The model under review builds one solid part; all positions refer to its coordinate system, in mm. A direction names the side the tool comes from. Round coordinates to 2 decimals unless told otherwise and drop trailing zeros. Order: outer loops, then holes, each group sorted by start corner. A loop starts at its lowest first (then second) coordinate and runs counter-clockwise, first axis right, second up. Notation, with made-up numbers: M -31,43 L 9,43 A27 ccw 9,78 Z; hole C -1.5,71 d11. An arc over 180 degrees is marked long. Answer as CSV lines item,"result". Start each with the question number.
Autodesk Inventor part; units mm, degrees
ref_plane "YZ Plane" through (0, 0, 0) normal (1, 0, 0) x (0, 1, 0)
ref_plane "XZ Plane" through (0, 0, 0) normal (0, 1, 0) x (-1, 0, 0)
ref_plane "XY Plane" through (0, 0, 0) normal (0, 0, 1) x (1, 0, 0)
sketch "Sketch1" plane through (0, 0, 0) normal (0, 1, 0) x (-1, 0, 0)
  line L0 (40, 20) -> (-40, 20) construction
  line L1 (-40, 20) -> (-40, -20) construction
  line L2 (-40, -20) -> (40, -20) construction
  line L3 (40, -20) -> (40, 20) construction
  line L4 (-40, 20) -> (40, -20) construction
  line L5 (0, 20) -> (0, -20) construction
  line L6 (-45, -25) -> (-45, 0)
  line L7 (-20, -25) -> (-45, -25)
  arc A0 (69.6915, -55.359) -> (90.0175, -26.0792) centre (75.7771, -37.8885) ccw
  circle A1 centre (75.7771, -37.8885) radius 8.5
  line L8 (69.6915, -55.359) -> (-15.0657, -25.8348)
  arc A2 (-15.0657, -25.8348) -> (-20, -25) centre (-20, -40) ccw
  arc A3 (90.0175, -26.0792) -> (69.6915, -55.359) centre (75.7771, -37.8885) ccw construction
  line L9 (-45, 0) -> (-45, 25)
  line L10 (-45, 25) -> (46.484, 25)
  line L11 (40, 0) -> (45, 0) construction
  line L12 (0, 20) -> (0, 25) construction
  line L13 (-40, 0) -> (-45, 0) construction
  line L14 (47.6585, 25) -> (48.4083, 24.0959) construction
  arc A4 (48.4083, 24.0959) -> (46.484, 25) centre (46.484, 22.5) ccw
  arc A5 (46.484, 25) -> (48.4083, 24.0959) centre (46.484, 22.5) ccw construction
  line L15 (48.4083, 24.0959) -> (90.0175, -26.0792)
  line L16 (46.484, 25) -> (47.6585, 25) construction
  point P0 (0, 0)
  point P1 (0, 0)
  point P2 (0, 0)
  dimension "d2" = 80
  dimension "d3" = 40
  dimension "d29" = 5
  dimension "d30" = 17
  dimension "d31" = 10
  dimension "d32" = 40
  dimension "d34" = 5
  dimension "d35" = 15
  dimension "d36" = 25
  dimension "d38" = 5
  dimension "d41" = 66.3579
extrude "Plate1" add sketch "Sketch1" along normal blind 3
fillet "Corner Round3" radius 6 2 edges at (45, 1.5, 25) (45, 1.5, -25)
equation "\"d34\" = d29"
equation "\"d6\" = Thickness"
properties part number "NDM-VOS Пятка под стойки" material "Stainless Steel"
Item 1: Consider section A-A (z = -32.5). State the section outline as (x, y) points, and give its area (3 significant figures).
Item 2: Wall thickness on probe 1 along Z at (x, y) = (38, 2.65); probe 2 along Z at (x, y) = (-74.5, 1.4); probe 3 along Z at (x, y) = (-82, 0.15): over which ranges is each line inside the solid? List them lowest first. Write a range as [from, to].
Item 3: Consider section B-B (y = 1.15). State the section outline as (x, z) points, and give its area (3 significant figures).
Item 4: Tool access review of faces 1 (the flat face through (45, 1, 0)), 2 (the flat face through (29, 1, -25)): name each direction out of +Z, -Z, +X, -X, +Y, -Y from which nothing blocks a thin tool from reaching the whole face with its end or side.
Item 5: The part is to be moulded in two halves that separate along Z. For faces 3 (the cylindrical face through (-91.164, 1.479, -48.16)), 4 (the cylindrical face through (-79.7, 1.48, -30.35)), 5 (the flat face through (-27.9, 1.5, -40.8)), say which applies: +Z half, -Z half, draft (parallel to the pull), parting line (faces both ways), or undercut.
Item 6: For pin 1 (19.5 mm diameter, centred on x = -75.78, z = -37.89, fed in from -Y); pin 2 (0.9 mm diameter, centred on x = 26.5, y = 2, fed in from -Z), all flat-tipped, find the tip position at first contact; note any pin that passes through.
Item 7: Consider section C-C (x = 22.5). State the section outline as (y, z) points.
Item 8: Consider section D-D (z = -2.5). State the section outline as (x, y) points.
Reported:
1,outline,"M -93.47,0 L -82.35,0 L -82.35,3 L -93.47,3 Z; M -69.2,0 L -4.07,0 L -4.07,3 L -69.2,3 Z"
1,area,"229 mm²"
2,probe 1,"z = [-25, 25]"
2,probe 2,"z = [-56.34, -46.29], [-29.48, -7.37]"
2,probe 3,"z = [-55.31, -43.68], [-32.1, -16.41]"
3,outline,"M -90.02,-26.08 A18.5 ccw -69.69,-55.36 L 15.07,-25.83 A15 cw 20,-25 L 39,-25 A6 ccw 45,-19 L 45,19 A6 ccw 39,25 L -46.48,25 A2.5 ccw -48.41,24.1 Z; hole C -75.78,-37.89 d17"
3,area,"7,430 mm²"
4,face 1,"+Z, -Z, +X, +Y, -Y"
4,face 2,"-Z, +X, +Y, -Y"
5,face 3,"parting line"
5,face 4,"undercut"
5,face 5,"-Z half"
6,pin 1,"stops at y = 0"
6,pin 2,"stops at z = -25"
7,outline,"M 0,-25 L 3,-25 L 3,25 L 0,25 Z"
8,outline,"M -70.46,0 L 45,0 L 45,3 L -70.46,3 Z"
